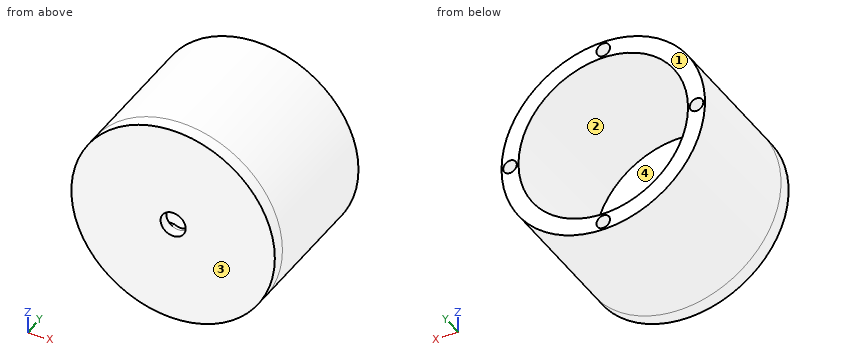
```python
from build123d import *

# Parameters (mm, degrees)
CROQUIS2_R              = 30
SALIENTE_EXTRUIR1_DEPTH = 4
CORTAR_EXTRUIR1_DEPTH   = 1
CROQUIS3_R              = 3.7
CORTAR_EXTRUIR2_DEPTH   = 3
CROQUIS5_W              = 5
CROQUIS5_H              = 80
CROQUIS6_R              = 2
CORTAR_EXTRUIR3_DEPTH   = 46
CROQUIS7_W              = 60
CROQUIS7_H              = 40
CORTAR_EXTRUIR4_DEPTH   = 30


with BuildPart() as part:
    # Croquis2 → Saliente-Extruir1 (new body)
    with BuildSketch(Plane(origin=(0, 0, 0), x_dir=(1, 0, 0), z_dir=(0, 1, 0))):
        Circle(CROQUIS2_R)
    extrude(amount=-SALIENTE_EXTRUIR1_DEPTH)

    # Croquis1 → Cortar-Extruir1 (cut)
    with BuildSketch(Plane(origin=(0, 0, 0), x_dir=(1, 0, 0), z_dir=(0, 1, 0))):
        with BuildLine():
            Line((18, -2.1), (18, 2.1))
            Line((18, 2.1), (1.92939966, 3.178620376))
            ThreePointArc((1.92939966, 3.178620376), (0, 3.718361271), (-1.92939966, 3.178620376))
            Line((-1.92939966, 3.178620376), (-18, 2.1))
            Line((-18, 2.1), (-18, -2.1))
            Line((-18, -2.1), (-1.92939966, -3.178620376))
            ThreePointArc((-1.92939966, -3.178620376), (0, -3.718361271), (1.92939966, -3.178620376))
            Line((1.92939966, -3.178620376), (18, -2.1))
        make_face()
    extrude(amount=-CORTAR_EXTRUIR1_DEPTH, mode=Mode.SUBTRACT)

    # Croquis3 → Cortar-Extruir2 (cut)
    with BuildSketch(Plane(origin=(0, -1, 0), x_dir=(1, 0, 0), z_dir=(0, 1, 0))):
        Circle(CROQUIS3_R)
    extrude(amount=-CORTAR_EXTRUIR2_DEPTH, mode=Mode.SUBTRACT)

    # Croquis5 → Revolución1 (revolve)
    with BuildSketch(Plane.XY):
        with Locations((27.5, 40)):
            Rectangle(CROQUIS5_W, CROQUIS5_H)
    revolve(axis=Axis((0, 80, 0), (0, -1, 0)))

    # Croquis6 → Cortar-Extruir3 (cut)
    with BuildSketch(Plane(origin=(0, 80, 0), x_dir=(1, 0, 0), z_dir=(0, 1, 0))):
        with Locations((27.5, 0)):
            Circle(CROQUIS6_R)
        with Locations((0, -27.5)):
            Circle(CROQUIS6_R)
        with Locations((-27.5, 0)):
            Circle(CROQUIS6_R)
        with Locations((0, 27.5)):
            Circle(CROQUIS6_R)
    extrude(amount=-CORTAR_EXTRUIR3_DEPTH, mode=Mode.SUBTRACT)

    # Croquis7 → Cortar-Extruir4 (cut)
    with BuildSketch(Plane.XY):
        with Locations((0, 60)):
            Rectangle(CROQUIS7_W, CROQUIS7_H)
    cortar_extruir4 = extrude(amount=-CORTAR_EXTRUIR4_DEPTH, mode=Mode.SUBTRACT)

    # Simetría1: Cortar-Extruir4 across plane
    add(cortar_extruir4.mirror(Plane.XY), mode=Mode.SUBTRACT)


solid = part.part
```
Can you work these out from the model? Positions are in its coordinate system, mm. Face numbers are marked on the shaded views. A direction names the side the tool comes from. Coordinates: 2 decimals unless noted, no trailing zeros. Order: outer loops, then holes, each group sorted by start corner. A loop starts at its lowest first (then second) coordinate and runs counter-clockwise, first axis right, second up.
1. Thinking about a two-plate mould opening in X: for the marked faces 1 and 2, which applies, +X half, -X half, draft (parallel to the pull), parting line (faces both ways), or undercut?
2. For the marked faces 3 and 4, which set-ups out of +Z, -Z, +X, -X, +Y, -Y let a thin tool reach every point of the face, with its end or its side?
3. I'm going to push flat-ended pins straight in: pin 1 (2 mm diameter, centred on x = 0, z = -27.5, fed in from +Y); pin 2 (12 mm diameter, centred on y = 1, z = -5.5, fed in from +X); pin 3 (1 mm diameter, centred on x = 13, y = 19.5, fed in from -Z); pin 4 (2 mm diameter, centred on x = 7.5, y = 35, fed in from -Z). Where does each tip first touch, or does it pass through?
4. If we section it at B-B (z = 0): Please give me the cut outline in (x, y), then the cut area to 3 significant figures.
5. If we section it at D-D (y = 32.5): Please give me the cut outline in (x, z), then the cut area to 3 significant figures.
6. If we section it at C-C (x = 24): Please give me the cut outline in (y, z).
7. I need wall thicknesses on line 1 (X direction, y = 29, z = 0); line 2 (Z direction, x = 0, y = -2); line 3 (X direction, y = 36, z = 1). Which ranges of each line are inside material? Lowest first, please.
Entries:
1. face 1: draft
1. face 2: undercut
2. face 3: +Z, -Z, +X, -X, -Y
2. face 4: +Y
3. pin 1: stops at y = 34
3. pin 2: stops at x = 30
3. pin 3: stops at z = -27.27
3. pin 4: stops at z = -29.29
4. outline: (-30, -4) - (-3.7, -4) - (-3.7, -1) - (-18, -1) - (-18, 0) - (-25, 0) - (-25, 40) - (-25.5, 40) - (-25.5, 34) - (-29.5, 34) - (-29.5, 40) - (-30, 40) - close; (3.7, -4) - (30, -4) - (30, 40) - (29.5, 40) - (29.5, 34) - (25.5, 34) - (25.5, 40) - (25, 40) - (25, 0) - (18, 0) - (18, -1) - (3.7, -1) - close
4. area: 534 mm2
5. outline: circle Ø60 at (0, 0); hole circle Ø50 at (0, 0)
5. area: 864 mm2
6. outline: (-4, -18) - (40, -18) - (40, -7) - (0, -7) - (0, 7) - (40, 7) - (40, 18) - (-4, 18) - close
7. line 1: x = -30 to -25, 25 to 30
7. line 2: z = -30 to -3.7, 3.7 to 30
7. line 3: x = -29.98 to -29.23, -25.77 to -24.98, 24.98 to 25.77, 29.23 to 29.98
